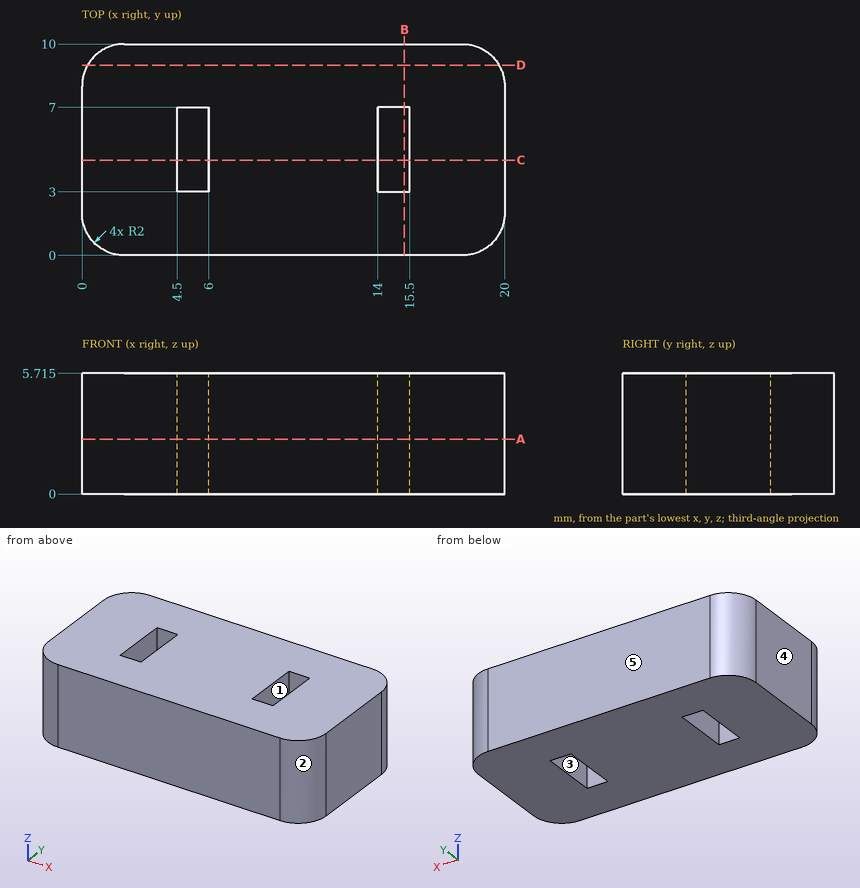
The figure shows three views and two pictorial views of one solid part (mm, origin at its lowest corner). Answer the questions. A direction names the side the tool comes from. Round coordinates to 2 decimals unless told otherwise and drop trailing zeros. Write each loop counter-clockwise with the first axis right and the second up, starting at its lowest first coordinate (ties: lowest second). Pieces come first, ordered by that corner, then holes. Notation, with made-up numbers: M 77,55 L 84,55 A10 ccw 84,62 Z; hole C 20.5,75.5 d6. An arc over 180 degrees is marked long. Use a Markdown table: item, result.
1) Consider line 1 (X direction, y = 6, z = 1.8); line 2 (Y direction, x = 5.25, z = 5.1); line 3 (X direction, y = 1.75, z = 4.25). Determine where each line is inside the solid, lowest interval first. Write a range as [from, to].
Taken from the geometry:
| item | result |
|---|---|
| line 1 | x = [0, 4.5], [6, 14], [15.5, 20] |
| line 2 | y = [0, 3], [7, 10] |
| line 3 | x = [0.02, 19.98] |
2) Which of the six approach directions +Z, -Z, +X, -X, +Y, -Y give full straight-line access (tool end or side, diameter ignored) to the marked faces 1 and 2?
Taken from the geometry:
| item | result |
|---|---|
| face 1 | +Z, -Z |
| face 2 | +Z, -Z, +X, -Y |
3) The part is cut by section B-B on x = 15.25. Give the vertices of the cut face in (y, z) (3 decimals), plus the area to 3 significant figures.
Taken from the geometry:
| item | result |
|---|---|
| outline | M 0,0 L 3,0 L 3,5.715 L 0,5.715 Z; M 7,0 L 10,0 L 10,5.715 L 7,5.715 Z |
| area | 34.3 mm2 |
4) The part is cut by section D-D on y = 9. Give the vertices of the cut face in (x, z) (3 decimals), plus the area to 3 significant figures.
Taken from the geometry:
| item | result |
|---|---|
| outline | M 0.268,0 L 19.732,0 L 19.732,5.715 L 0.268,5.715 Z |
| area | 111 mm2 |
5) The part is cut by section A-A on z = 2.6. Give the vertices of the cut face in (x, y).
Taken from the geometry:
| item | result |
|---|---|
| outline | M 0,2 A2 ccw 2,0 L 18,0 A2 ccw 20,2 L 20,8 A2 ccw 18,10 L 2,10 A2 ccw 0,8 Z; hole M 4.5,3 L 6,3 L 6,7 L 4.5,7 Z; hole M 14,3 L 15.5,3 L 15.5,7 L 14,7 Z |
6) The part is cut by section C-C on y = 4.5. Give the vertices of the cut face in (x, z) (3 decimals), plus the area to 3 significant figures.
Taken from the geometry:
| item | result |
|---|---|
| outline | M 0,0 L 4.5,0 L 4.5,5.715 L 0,5.715 Z; M 6,0 L 14,0 L 14,5.715 L 6,5.715 Z; M 15.5,0 L 20,0 L 20,5.715 L 15.5,5.715 Z |
| area | 97.2 mm2 |
7) Determine the mould class of the marked faces 3, 4 and 5 for opening direction Y: pulls with the +Y half, pulls with the -Y half, needs draft (parallel to the pull), parting line crosses it, or undercut.
Taken from the geometry:
| item | result |
|---|---|
| face 3 | undercut |
| face 4 | needs draft |
| face 5 | pulls with the +Y half |
8) A flat-ended cylindrical pin translates along its axis: pin 1 (1 mm diameter, centred on x = 11.5, y = 4.5, fed in from -Z). Find the tip coordinate at first contact, or state that the pin passes through.
Taken from the geometry:
| item | result |
|---|---|
| pin 1 | stops at z = 0 |
